Can you work these out from the drawing? Everything is in mm from the part's minimum corner. Coordinates: 2 decimals unless noted, no trailing zeros. Order: outer loops, then holes, each group sorted by start corner. A loop starts at its lowest first (then second) coordinate and runs counter-clockwise, first axis right, second up. Notation, with made-up numbers: (51, -40) - (58, -40) arc R14 cw to (58, -16) - close; hole circle Ø5 at (7.25, 50). An arc over 180 degrees is marked (long way). Use a Markdown table: item, result. Add a question column.
(1) I want a section at A-A (y = 95). List the corners of the cut face in (x, z) for me.
(2) If I drill on L1, parallel to Z at x = 71.75, y = 10 (1 decimal); L2, parallel to Y at x = 77, z = 10 (1 decimal); L3, parallel to Y at x = 65.5, z = 189, over which ranges is the centre line in solid material (lowest first)? Write a range as [from, to].
(3) I want a section at B-B (x = 75). List the corners of the cut face in (y, z) for me.
(4) For pin 1 Ø7 at (y, z) = (10, 370) entering from +X; pin 2 Ø22 at (x, z) = (70.5, 307.5) entering from +Y; pin 3 Ø1 at (x, y) = (100, 73.5) entering from -Z, each with a flat end and sliding along its axis, tell me the tip position at first contact or that it passes through.
(5) I want a section at C-C (z = 287). List the corners of the cut face in (x, y) for me.
(6) I want a section at D-D (x = 50.5). List the corners of the cut face in (y, z) for me (1 decimal).
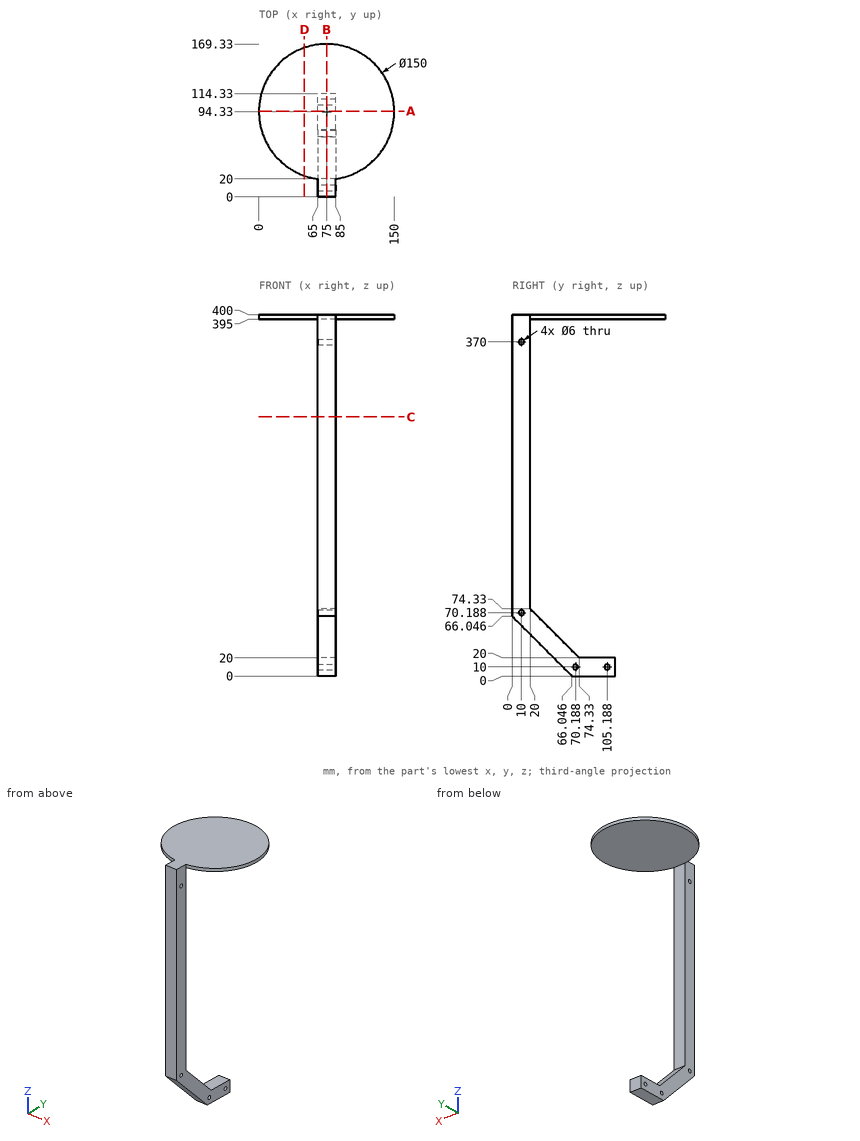
Answers follow:
| question | item | result |
|---|---|---|
| 1 | outline | (0, 395) - (150, 395) - (150, 400) - (0, 400) - close; (65, 0) - (85, 0) - (85, 20) - (65, 20) - close |
| 2 | L1 | z = [56, 67.2], [73.2, 367], [373, 400] |
| 2 | L2 | y = [56, 67.2], [73.2, 102.2], [108.2, 114.3] |
| 2 | L3 | y = [0, 20] |
| 3 | outline | (0, 66.05) - (66.05, 0) - (114.33, 0) - (114.33, 20) - (74.33, 20) - (20, 74.33) - (20, 395) - (169.33, 395) - (169.33, 400) - (0, 400) - close; hole circle Ø6 at (10, 70.19); hole circle Ø6 at (10, 370); hole circle Ø6 at (70.19, 10); hole circle Ø6 at (105.19, 10) |
| 4 | pin 1 | stops at x = 85 |
| 4 | pin 2 | stops at y = 20 |
| 4 | pin 3 | stops at z = 395 |
| 5 | outline | (65, 0) - (85, 0) - (85, 20) - (65, 20) - close |
| 6 | outline | (23.4, 395) - (165.2, 395) - (165.2, 400) - (23.4, 400) - close |
